The figure shows three views and two pictorial views of one solid part (mm, origin at its lowest corner). Answer the questions. A direction names the side the tool comes from. Round coordinates to 2 decimals unless told otherwise and drop trailing zeros. Write each loop counter-clockwise with the first axis right and the second up, starting at its lowest first coordinate (ties: lowest second). Pieces come first, ordered by that corner, then holes.
Item 1: This flat-tipped pin is pushed along its axis until it touches: pin 1 (4.5 mm diameter, centred on y = 43, z = 8, fed in from -X). Where does it stop, or does it pass through?
Item 2: A tool of negligible diameter and unlimited length cuts with its end or side. For the marked faces 1 and 2, from which of +Z, -Z, +X, -X, +Y, -Y can it reach the whole face along a straight path? Write none if from no direction.
Item 3: For a pull along Z with two mould halves and no side action, classify the marked faces 3, 4 and 5 as +Z half, -Z half, draft (parallel to the pull), parting line (faces both ways), or undercut.
Item 4: Find section D-D on y = 27.5. Give the vertices of the cut face in (x, z), then the cut area to 3 significant figures.
Item 5: Find section B-B on y = 43. Give the vertices of the cut face in (x, z).
Item 6: Find section C-C on x = 5.5. Give the vertices of the cut face in (y, z).
Item 7: Find the intervals of material crossed by probe 1 along Y at (x, z) = (13.35, 8); probe 2 along Z at (x, y) = (9.5, 14); probe 3 along X at (y, z) = (16.5, 4), in increasing order.
Item 8: Find section A-A on z = 8. Give the vertices of the cut face in (x, y), then the cut area to 3 significant figures.
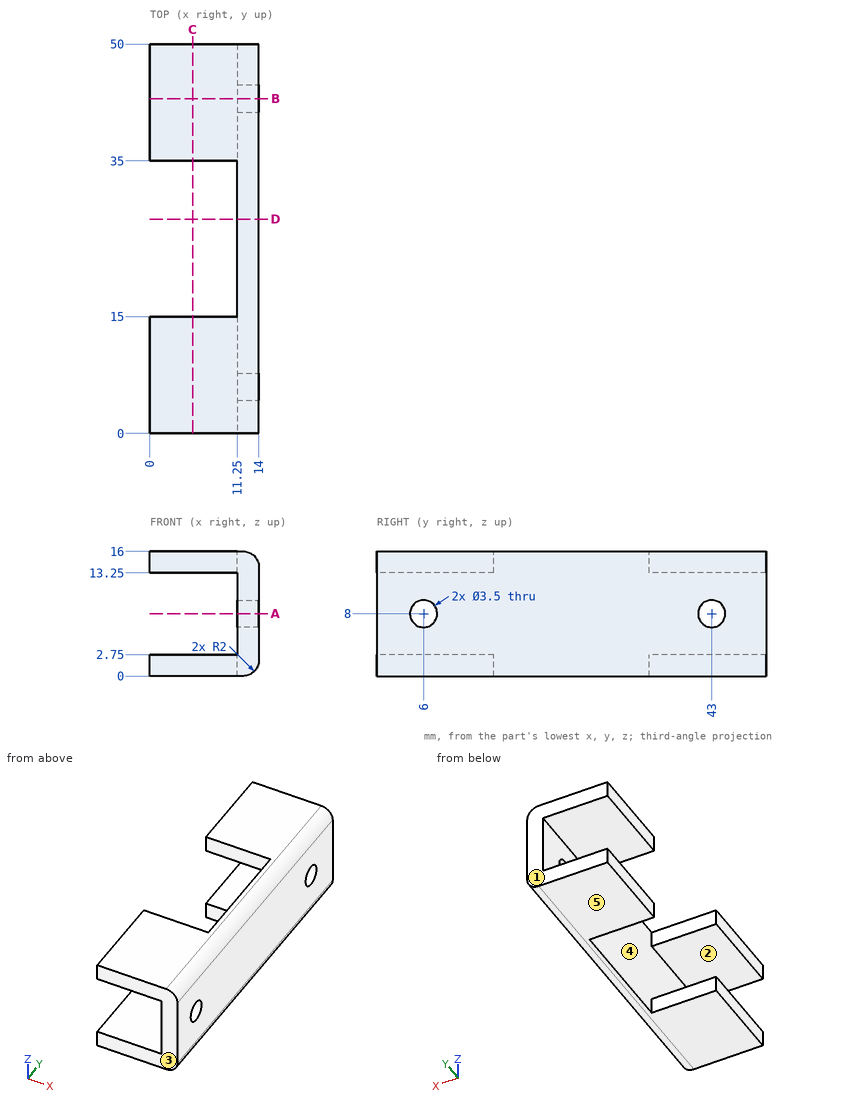
Check values:
1. pin 1: stops at x = 11.25
2. face 1: +Z, -Z, +X, -X, +Y
2. face 2: -X, +Y, -Y
3. face 3: draft
3. face 4: undercut
3. face 5: -Z half
4. outline: (11.25, 0) - (12, 0) arc R2 ccw to (14, 2) - (14, 14) arc R2 ccw to (12, 16) - (11.25, 16) - close
4. area: 42.3 mm2
5. outline: (0, 0) - (12, 0) arc R2 ccw to (14, 2) - (14, 6.25) - (11.25, 6.25) - (11.25, 2.75) - (0, 2.75) - close; (0, 13.25) - (11.25, 13.25) - (11.25, 9.75) - (14, 9.75) - (14, 14) arc R2 ccw to (12, 16) - (0, 16) - close
6. outline: (0, 0) - (15, 0) - (15, 2.75) - (0, 2.75) - close; (0, 13.25) - (15, 13.25) - (15, 16) - (0, 16) - close; (35, 0) - (50, 0) - (50, 2.75) - (35, 2.75) - close; (35, 13.25) - (50, 13.25) - (50, 16) - (35, 16) - close
7. probe 1: y = 0 to 4.25, 7.75 to 41.25, 44.75 to 50
7. probe 2: z = 0 to 2.75, 13.25 to 16
7. probe 3: x = 11.25 to 14
8. outline: (11.25, 0) - (14, 0) - (14, 4.25) - (11.25, 4.25) - close; (11.25, 7.75) - (14, 7.75) - (14, 41.25) - (11.25, 41.25) - close; (11.25, 44.75) - (14, 44.75) - (14, 50) - (11.25, 50) - close
8. area: 118 mm2
